Study the drawing (mm; zero at the part's minimum x, y, z) and answer. A direction names the side the tool comes from. Give positions to 0.01 mm unless a question says otherwise; leave off trailing zeros. Write each loop counter-clockwise with the first axis right and the second up, starting at its lowest first coordinate (ties: lowest second). Pieces come first, ordered by that corner, then holes.
1) A tool of negligible diameter and unlimited length cuts with its end or side. For the marked faces 1, 2, 3 and 4, from which of +Z, -Z, +X, -X, +Y, -Y can it reach the whole face along a straight path? Write none if from no direction.
2) Find section D-D (x = 17). Determine the outline of the cut face in (y, z).
3) Find section C-C (y = 14). Determine the outline of the cut face in (x, z), plus the area to 3 significant figures.
4) Straight lines are drawn through the part: probe 1 along Z at (x, y) = (51.2, 13.85); probe 2 along X at (y, z) = (13.95, 5); probe 3 along Z at (x, y) = (52.5, 13). For each, find the intervals that lie inside material, in ascending order.
5) Find section A-A (z = 5). Determine the outline of the cut face in (x, y), plus the area to 3 significant figures.
6) Given pin 1 Ø2 at (x, z) = (2.5, 7.5) entering from +Y; pin 2 Ø2 at (x, z) = (51.5, 7.5) entering from -Y; pin 3 Ø6 at (y, z) = (24, 11.5) entering from -X, each flat-ended and moving along its own axis, determine where each tip first touches the part or whether it passes through.
7) Find section B-B (x = 51.2). Determine the outline of the cut face in (y, z), plus the area to 3 significant figures.
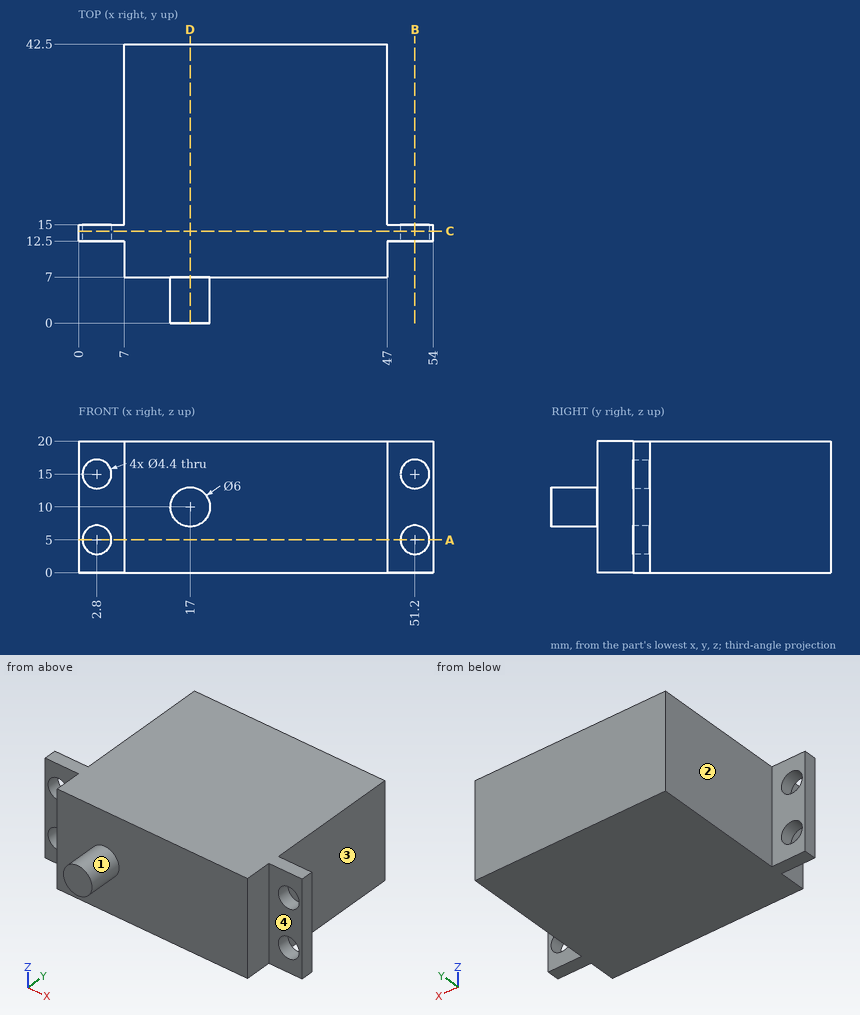
Results:
1. face 1: -Y
1. face 2: +Z, -Z, -X, +Y
1. face 3: +Z, -Z, +X, +Y
1. face 4: +Z, -Z, +X, -Y
2. outline: (0, 7) - (7, 7) - (7, 0) - (42.5, 0) - (42.5, 20) - (7, 20) - (7, 13) - (0, 13) - close
3. outline: (0, 0) - (54, 0) - (54, 20) - (0, 20) - close; hole circle Ø4.4 at (2.8, 5); hole circle Ø4.4 at (2.8, 15); hole circle Ø4.4 at (51.2, 5); hole circle Ø4.4 at (51.2, 15)
3. area: 1,020 mm2
4. probe 1: z = 0 to 2.8, 7.2 to 12.8, 17.2 to 20
4. probe 2: x = 0 to 0.6, 5 to 49, 53.4 to 54
4. probe 3: z = 0 to 3.23, 6.77 to 13.23, 16.77 to 20
5. outline: (0, 12.5) - (0.6, 12.5) - (0.6, 15) - (0, 15) - close; (5, 12.5) - (7, 12.5) - (7, 7) - (47, 7) - (47, 12.5) - (49, 12.5) - (49, 15) - (47, 15) - (47, 42.5) - (7, 42.5) - (7, 15) - (5, 15) - close; (53.4, 12.5) - (54, 12.5) - (54, 15) - (53.4, 15) - close
5. area: 1,430 mm2
6. pin 1: stops at y = 15
6. pin 2: stops at y = 12.5
6. pin 3: stops at x = 7
7. outline: (12.5, 0) - (15, 0) - (15, 2.8) - (12.5, 2.8) - close; (12.5, 7.2) - (15, 7.2) - (15, 12.8) - (12.5, 12.8) - close; (12.5, 17.2) - (15, 17.2) - (15, 20) - (12.5, 20) - close
7. area: 28.0 mm2
